Drawing for the job (mm, zero at the part's lowest x, y, z). A direction names the side the tool comes from. Round coordinates to 2 decimals unless told otherwise and drop trailing zeros. Order: outer loops, then holes, each group sorted by start corner. A loop starts at its lowest first (then second) coordinate and runs counter-clockwise, first axis right, second up. Notation, with made-up numbers: (8.25, 4) - (16.25, 4) arc R35 ccw to (16.25, 43) - close; hole circle Ø7 at (22.25, -4.5). An arc over 180 degrees is marked (long way). Put each result on its own line as item: value. Start each with the question number.
Item 1: Probe probe 1 along Y at (x, z) = (51, 11.25); probe 2 along X at (y, z) = (14, 4.25); probe 3 along X at (y, z) = (17, 2). List the from-to ranges inside material, lowest first.
Item 2: Mould opens along X. For the marked faces 1, 2 and 3 say: pulls with the +X half, pulls with the -X half, needs draft (parallel to the pull), parting line crosses it, or undercut.
Item 3: Saw through at D-D on y = 3.5. List the corners of the cut face in (x, z), plus the area to 3 significant figures.
Item 4: Pin check, flat tips, straight feed: pin 1 Ø6.5 at (y, z) = (8.5, 7.5) entering from -X; pin 2 Ø4 at (y, z) = (10, 5.5) entering from +X; pin 3 Ø6.5 at (x, z) = (47.5, 5.5) entering from +Y. Stop position of each tip, or through.
Item 5: Saw through at B-B on z = 3.5. List the corners of the cut face in (x, y).
Item 6: Which spindle directions (+Z, -Z, +X, -X, +Y, -Y) get a long thin tool onto all of the face, cutting with end or side? Do the marked faces 4 and 5. Say none if no direction does.
Item 7: Saw through at C-C on x = 56. List the corners of the cut face in (y, z).
Item 8: Saw through at A-A on y = 14.25. List the corners of the cut face in (x, z).
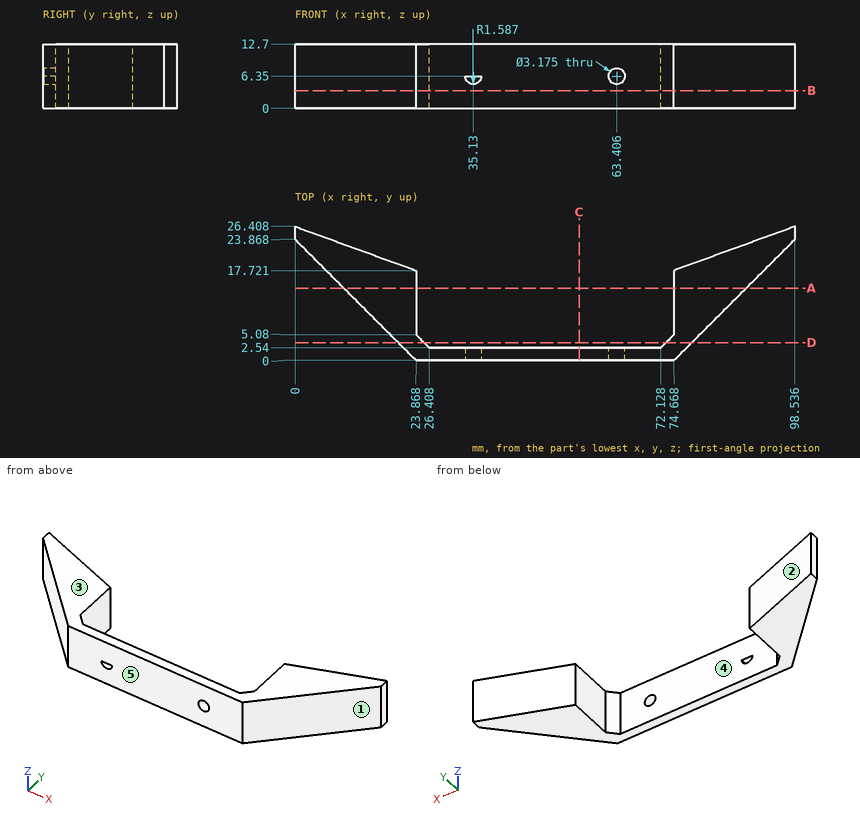
Results found:
1. probe 1: y = 0 to 2.54
1. probe 2: x = 9.87 to 23.87, 74.67 to 88.67
1. probe 3: x = 6.87 to 23.87, 74.67 to 91.67
2. face 1: pulls with the +X half
2. face 2: undercut
2. face 3: needs draft
3. outline: (20.37, 0) - (25.45, 0) - (25.45, 12.7) - (20.37, 12.7) - close; (73.09, 0) - (78.17, 0) - (78.17, 12.7) - (73.09, 12.7) - close
3. area: 129 mm²
4. pin 1: stops at x = 12.12
4. pin 2: stops at x = 86.67
4. pin 3: stops at y = 2.54
5. outline: (0, 23.87) - (23.87, 0) - (74.67, 0) - (98.54, 23.87) - (98.54, 26.41) - (74.67, 17.72) - (74.67, 5.08) - (72.13, 2.54) - (26.41, 2.54) - (23.87, 5.08) - (23.87, 17.72) - (0, 26.41) - close
6. face 4: +Z, -Z, +Y
6. face 5: +Z, -Z, +X, -X, -Y
7. outline: (0, 0) - (2.54, 0) - (2.54, 12.7) - (0, 12.7) - close
8. outline: (9.62, 0) - (23.87, 0) - (23.87, 12.7) - (9.62, 12.7) - close; (74.67, 0) - (88.92, 0) - (88.92, 12.7) - (74.67, 12.7) - close
